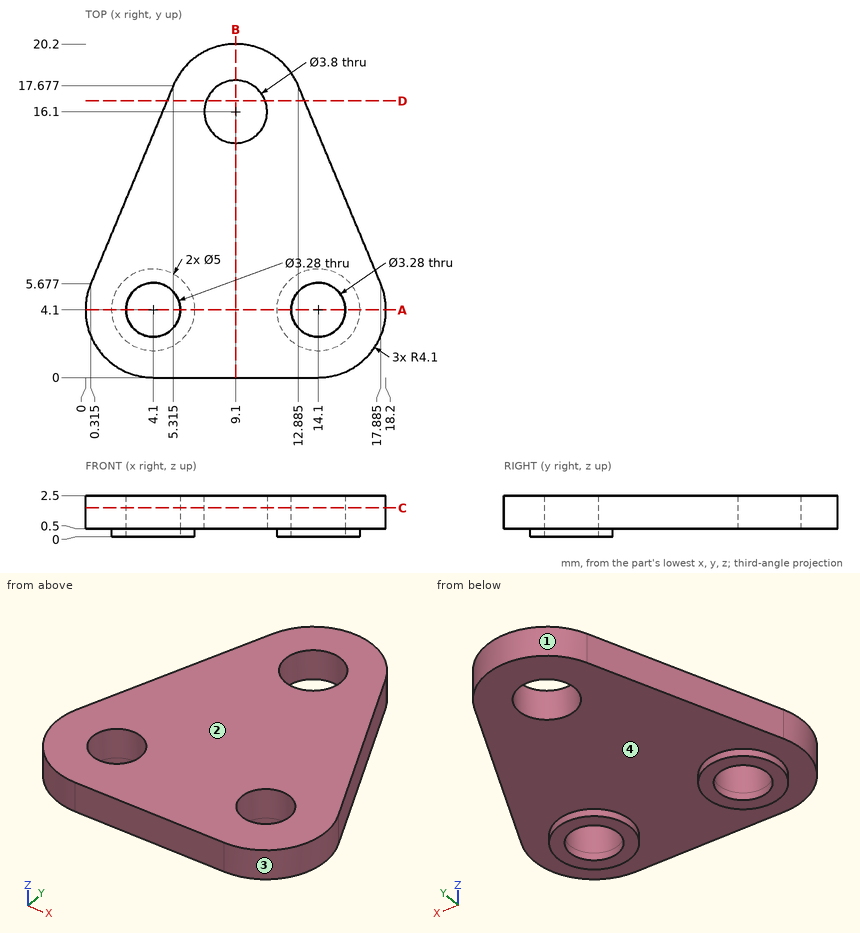
The figure shows three views and two pictorial views of one solid part (mm, origin at its lowest corner). Answer the questions. Coordinates: 2 decimals unless noted, no trailing zeros. Loops run counter-clockwise (first coordinate to the right, second up) from the corner with the lowest first, then second, coordinate; pieces in that order, holes last.
(1) Consider line 1 along Y through (x, z) = (4.1, 0.2); line 2 along X through (y, z) = (3.25, 1.35); line 3 along Z through (x, y) = (10.75, 9). Determine where each line is inside the solid, lowest interval first.
Solution:
line 1: y = 1.6 to 2.46, 5.74 to 6.6
line 2: x = 0.09 to 2.7, 5.5 to 12.7, 15.5 to 18.11
line 3: z = 0.5 to 2.5
(2) The part is cut by section C-C (z = 1.75). Determine the outline of the cut face in (x, y) (1 decimal), and give its area (3 significant figures).
Solution:
outline: (0.3, 5.7) arc R4.1 ccw to (4.1, 0) - (14.1, 0) arc R4.1 ccw to (17.9, 5.7) - (12.9, 17.7) arc R4.1 ccw to (5.3, 17.7) - close; hole circle Ø3.3 at (4.1, 4.1); hole circle Ø3.8 at (9.1, 16.1); hole circle Ø3.3 at (14.1, 4.1)
area: 232 mm2
(3) The part is cut by section A-A (y = 4.1). Determine the outline of the cut face in (x, z).
Solution:
outline: (0, 0.5) - (1.6, 0.5) - (1.6, 0) - (2.46, 0) - (2.46, 2.5) - (0, 2.5) - close; (5.74, 0) - (6.6, 0) - (6.6, 0.5) - (11.6, 0.5) - (11.6, 0) - (12.46, 0) - (12.46, 2.5) - (5.74, 2.5) - close; (15.74, 0) - (16.6, 0) - (16.6, 0.5) - (18.2, 0.5) - (18.2, 2.5) - (15.74, 2.5) - close
(4) Flat-ended cylindrical pins translate along their axes: pin 1 Ø4.5 at (x, y) = (4.1, 4.1) entering from -Z; pin 2 Ø4 at (x, y) = (4, 11.5) entering from -Z. Find the tip coordinate at first contact, or state that the pin passes through.
Solution:
pin 1: stops at z = 0
pin 2: stops at z = 0.5
(5) The part is cut by section D-D (y = 16.75). Determine the outline of the cut face in (x, z) (1 decimal).
Solution:
outline: (4.9, 0.5) - (7.3, 0.5) - (7.3, 2.5) - (4.9, 2.5) - close; (10.9, 0.5) - (13.3, 0.5) - (13.3, 2.5) - (10.9, 2.5) - close
(6) The mould has two halves that part along X. Classify the marked faces 1, 2, 3 and 4: released by +X, released by -X, zero draft, split by the parting line, or undercut.
Solution:
face 1: split by the parting line
face 2: zero draft
face 3: released by +X
face 4: undercut
(7) The part is cut by section B-B (x = 9.1). Determine the outline of the cut face in (y, z).
Solution:
outline: (0, 0.5) - (14.2, 0.5) - (14.2, 2.5) - (0, 2.5) - close; (18, 0.5) - (20.2, 0.5) - (20.2, 2.5) - (18, 2.5) - close
